Geometry check sheet. Reference: the model listing, model coordinates, mm. Face numbers are marked on the shaded views. A direction names the side the tool comes from. Give positions to 0.01 mm unless a question says otherwise; leave off trailing zeros. Order: outer loops, then holes, each group sorted by start corner. A loop starts at its lowest first (then second) coordinate and runs counter-clockwise, first axis right, second up.
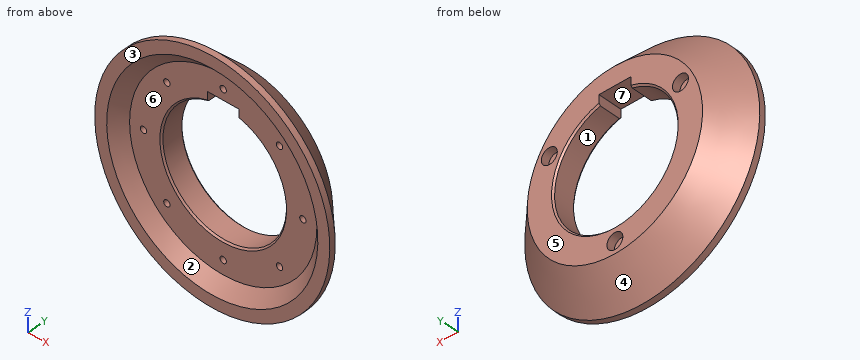
from build123d import *

# Parameters (mm, degrees)
CHAMFER_1_SIZE           = 2
SKETCH_2_R               = 10
CUT_EXTRUDE_1_DEPTH      = 10
PATTERN_CIRCULAR_1_COUNT = 3
CUT_EXTRUDE_2_DEPTH      = 214.395173329
CUT_EXTRUDE_2_DEPTH_BACK = 214.395173329
SKETCH_3_W               = 40
SKETCH_3_H               = 24.854018102
SKETCH_4_R               = 4
CUT_EXTRUDE_3_DEPTH      = 8
PATTERN_CIRCULAR_2_COUNT = 8


with BuildPart() as part:
    # Эскиз1 → Повернуть1 (revolve)
    with BuildSketch(Plane.XY, mode=Mode.PRIVATE) as revolve_1_sk:
        Polygon((77.5, 30), (77.5, 0), (117.5, 0), (132.5, -15), (147.5, -15), (147.5, -7.5), (110, 30), align=None)
    revolve(revolve_1_sk.sketch.rotate(Axis((0, 107.750556793, 0), (0, -1, 0)), 90), axis=Axis((0, 107.750556793, 0), (0, -1, 0)))

    # Фаска1
    chamfer_1_edges = [part.edges().sort_by_distance(p)[0] for p in [
        (0, 0, -77.5),
        (0, 30, -77.5),
    ]]
    chamfer(chamfer_1_edges, length=CHAMFER_1_SIZE)

    # Эскиз2 → Вырез-Вытянуть1 (cut)
    with BuildSketch(Plane(origin=(0, 30, 0), x_dir=(1, 0, 0), z_dir=(0, 1, 0))):
        with Locations(Location((0, 95, 0), (0, 0, 270))):
            Circle(SKETCH_2_R)
    cut_extrude_1 = extrude(amount=-CUT_EXTRUDE_1_DEPTH, mode=Mode.SUBTRACT)

    # Круговой массив1: Вырез-Вытянуть1 ×3 about axis
    pattern_circular_1_axis = Axis((0, 0, 0), (0, 1, 0))
    for i in range(1, PATTERN_CIRCULAR_1_COUNT):
        add(cut_extrude_1.rotate(pattern_circular_1_axis, i * 360 / PATTERN_CIRCULAR_1_COUNT), mode=Mode.SUBTRACT)

    # Эскиз3 → Вырез-Вытянуть2 (cut, two sides: drawn at the far end of the back side and taken through both)
    with BuildSketch(Plane(origin=(0, 30, 0), x_dir=(1, 0, 0), z_dir=(0, 1, 0)).offset(-CUT_EXTRUDE_2_DEPTH_BACK)):
        with Locations((0, -74.472990949)):
            Rectangle(SKETCH_3_W, SKETCH_3_H)
    extrude(amount=CUT_EXTRUDE_2_DEPTH + CUT_EXTRUDE_2_DEPTH_BACK, mode=Mode.SUBTRACT)

    # Эскиз4 → Вырез-Вытянуть3 (cut)
    with BuildSketch(Plane.XZ):
        with Locations(Location((0, 100, 0), (0, 0, 270))):
            Circle(SKETCH_4_R)
    cut_extrude_3 = extrude(amount=-CUT_EXTRUDE_3_DEPTH, mode=Mode.SUBTRACT)

    # Круговой массив2: Вырез-Вытянуть3 ×8 about axis
    pattern_circular_2_axis = Axis((0, 0, 0), (0, 1, 0))
    for i in range(1, PATTERN_CIRCULAR_2_COUNT):
        add(cut_extrude_3.rotate(pattern_circular_2_axis, i * 360 / PATTERN_CIRCULAR_2_COUNT), mode=Mode.SUBTRACT)


solid = part.part
Item 1: Set-up check for the marked faces 5, 6 and 7: record each of +Z, -Z, +X, -X, +Y, -Y from which the full face is reachable in a straight line by a thin tool's end or side.
Reported:
face 5: +Z, -Z, +X, -X, +Y
face 6: -Y
face 7: +Y, -Y
Item 2: Scan lines: L1, parallel to Z at x = -25, y = 6; L2, parallel to X at y = 25, z = -57; L3, parallel to Z at x = 52, y = -5.5. Record each from-to range of solid material in increasing order.
Reported:
L1: z = -131.65 to -73.36, 73.36 to 131.65
L2: x = -99.88 to -52.51, 52.51 to 99.88
L3: z = -135.89 to -111.47, 111.47 to 135.89
Item 3: Sectioned sample at A-A (z = 0). Enter the section's corners in (x, y), and give its area (3 significant figures).
Reported:
outline: (-147.5, -15) - (-132.5, -15) - (-117.5, 0) - (-104, 0) - (-104, 8) - (-96, 8) - (-96, 0) - (-79.5, 0) - (-77.5, 2) - (-77.5, 28) - (-79.5, 30) - (-110, 30) - (-147.5, -7.5) - close; (77.5, 2) - (79.5, 0) - (96, 0) - (96, 8) - (104, 8) - (104, 0) - (117.5, 0) - (132.5, -15) - (147.5, -15) - (147.5, -7.5) - (110, 30) - (79.5, 30) - (77.5, 28) - close
area: 3,330 mm2
Item 4: Draft check along Z on the marked faces 1, 2, 3 and 4. Enter one of: released by +Z, released by -Z, zero draft, split by the parting line, or undercut.
Reported:
face 1: undercut
face 2: undercut
face 3: zero draft
face 4: split by the parting line
Item 5: Sectioned sample at C-C (y = 16.5). Enter the section's corners in (x, z), and give its area (3 significant figures).
Reported:
outline: circle Ø247 at (0, 0); hole (-20, 74.87) arc R77.5 ccw (long way) to (20, 74.87) - (20, 86.9) - (-20, 86.9) - close
area: 28,600 mm2
Item 6: Sectioned sample at D-D (y = -11). Enter the section's corners in (x, z), and give its area (3 significant figures).
Reported:
outline: circle Ø295 at (0, 0); hole circle Ø257 at (0, 0)
area: 16,500 mm2
Item 7: Gauge pin test, flat ends, axial feed: pin 1 (4 mm diameter, centred on x = 69.5, z = 70, fed in from -Y); pin 2 (6.5 mm diameter, centred on x = 0, z = -100, fed in from +Y); pin 3 (5 mm diameter, centred on y = 24.5, z = 75, fed in from +X). Record the tip position at first contact, or that the pin passes through.
Reported:
pin 1: stops at y = 8
pin 2: stops at y = 20
pin 3: stops at x = 91.69
Item 8: Sectioned sample at B-B (x = 0). Enter the section's corners in (y, z), and give its area (3 significant figures).
Reported:
outline: (-15, -147.5) - (-7.5, -147.5) - (30, -110) - (30, -105) - (20, -105) - (20, -85) - (30, -85) - (30, -79.5) - (28, -77.5) - (2, -77.5) - (0, -79.5) - (0, -96) - (8, -96) - (8, -104) - (0, -104) - (0, -117.5) - (-15, -132.5) - close; (-15, 132.5) - (0, 117.5) - (0, 104) - (8, 104) - (8, 96) - (0, 96) - (0, 86.9) - (30, 86.9) - (30, 110) - (-7.5, 147.5) - (-15, 147.5) - close
area: 2,850 mm2
